Autodesk Inventor part; units mm, degrees
ref_plane "YZ Plane" through (0, 0, 0) normal (1, 0, 0) x (0, 1, 0)
ref_plane "XZ Plane" through (0, 0, 0) normal (0, 1, 0) x (-1, 0, 0)
ref_plane "XY Plane" through (0, 0, 0) normal (0, 0, 1) x (1, 0, 0)
sketch "Sketch1" plane through (0, 0, 0) normal (0, 1, 0) x (-1, 0, 0)
  line L0 (0, 0) -> (-200, 0)
  line L1 (-200, 0) -> (-200, -190)
  line L2 (-200, -190) -> (0, -190)
  line L3 (0, -190) -> (0, 0)
  line L4 (-65, 0) -> (-135, 0)
  line L5 (-135, 0) -> (-135, -5)
  line L6 (-135, -5) -> (-65, -5)
  line L7 (-65, -5) -> (-65, 0)
  line L8 (-200, -95) -> (0, -95) construction
  line L9 (-65, -190) -> (-135, -190)
  line L10 (-135, -190) -> (-135, -185)
  line L11 (-135, -185) -> (-65, -185)
  line L12 (-65, -185) -> (-65, -190)
  line L13 (-200, -215) -> (-200, -15)
  dimension "d0" = 200
  dimension "d2" = 70
  dimension "d3" = 5
  dimension "d11" = 0
  dimension "d13" = 190
extrude "Extrusion1" add sketch "Sketch1" along normal blind 5 contours L3 L2 L12 L11 L10 L1 L0 L5 L6 L7
sketch "Sketch2" plane through (0, 5, 0) normal (0, 1, 0) x (1, 0, 0)
  line L0 (0, 0) -> (65, 0)
  line L1 (135, 0) -> (200, 0)
  line L2 (65, 0) -> (65, 5)
  line L3 (0, 190) -> (0, 0)
  line L4 (0, 95) -> (200, 95)
  point P0 (95, 20)
  point P1 (105, 20)
  point P2 (95, 170)
  point P3 (105, 170)
  dimension "d22" = 20
  dimension "d23" = 10
  dimension "d24" = 20
  dimension "d25" = 30
hole "Hole1" at (95, 5, -20) at (105, 5, -20) at (95, 5, -170) at (105, 5, -170) direction (0, -1, 0) diameter 4 end through all
sketch "Sketch5" plane through (0, 5, 0) normal (0, 1, 0) x (1, 0, 0)
  line L0 (200, 0) -> (200, 190)
  line L1 (200, 190) -> (135, 190)
  point P0 (0, 0)
  point P1 (180, 90)
  point P2 (180, 100)
  dimension "d51" = 20
  dimension "d52" = 20
  dimension "d53" = 10
  dimension "d54" = 90
hole "Hole4" at (180, 5, -90) at (180, 5, -100) direction (0, -1, 0) diameter 4 end through all
sketch "Sketch6" plane through (0, 5, 0) normal (0, 1, 0) x (1, 0, 0)
  line L0 (0, 190) -> (0, 0)
  point P0 (45, 85.6926)
  point P1 (45, 107.7076)
  dimension "d62" = 45
  dimension "d63" = 45
  dimension "d64" = 22.015
hole "Hole5" at (45, 5, -85.6926) at (45, 5, -107.7076) direction (0, -1, 0) diameter 3 end through all
properties part number "top"
Source: CAD feature listing. Evaluate the final solid. Frame: model axes, mm. A direction names the side the tool comes from. Coordinates: 2 decimals unless noted, no trailing zeros. Loops run counter-clockwise (first coordinate to the right, second up) from the corner with the lowest first, then second, coordinate; pieces in that order, holes last. Notation, with made-up numbers: (28, 25.5) - (75, 25.5) arc R15 ccw to (75, 52.5) - close; hole circle Ø3 at (62.25, -12.5). An arc over 180 degrees is marked (long way). One line per item, written item: value. Start each with the question number.
1. Set-up query: faces 4 (the flat face through (65, 2, -3)), 5 (the flat face through (168, 2, -190)), 6 (the flat face through (135, 2, -188)). Return all of +Z, -Z, +X, -X, +Y, -Y with unobstructed straight access to the full face (end or side cutting, diameter ignored); none if empty.
2. Mould query, pull axis X, two halves, no side actions, for faces 1 (the flat face through (0, 2, -96)), 2 (the flat face through (65, 2, -187)), 3 (the flat face through (101, 0, -94)). Classes: pulls with the +X half, pulls with the -X half, needs draft (parallel to the pull), parting line crosses it, or undercut.
3. Ray query, L1, parallel to X at y = 2.75, z = -20; L2, parallel to Z at x = 105, y = 2.6; L3, parallel to Z at x = 45, y = 1.2. Return the intervals inside material, ascending.
4. Section B-B (x = 69.5). Return the cut outline in (y, z), and give its area (3 significant figures).
5. Section A-A (y = 1.05). State how many separate pieces and enclosed holes the cut face has, and give its area (3 significant figures).
6. Contact query for flat-ended pins moving along their axis: P1, Ø2.5, axis at x = 105, z = -20, coming from the -Y side; P2, Ø2, axis at x = 130.5, y = 4, coming from the -Z side. Output: stop coordinate, or through.
Verdict:
1. face 4: +Z, +Y, -Y
1. face 5: -Z, +X, -X, +Y, -Y
1. face 6: -Z, +Y, -Y
2. face 1: pulls with the -X half
2. face 2: undercut
2. face 3: needs draft
3. L1: x = 0 to 93, 97 to 103, 107 to 200
3. L2: z = -185 to -172, -168 to -22, -18 to -5
3. L3: z = -190 to -109.21, -106.21 to -87.19, -84.19 to 0
4. outline: (0, -185) - (5, -185) - (5, -5) - (0, -5) - close
4. area: 900 mm2
5. separate pieces: 1
5. enclosed holes: 8
5. area: 37,200 mm2
6. P1: passes through
6. P2: stops at z = -185
